Design review of the part built by this model. Coordinates are the model's own, in mm. A direction names the side the tool comes from. Round coordinates to 2 decimals unless told otherwise and drop trailing zeros. Write each loop counter-clockwise with the first axis right and the second up, starting at its lowest first coordinate (ties: lowest second). Pieces come first, ordered by that corner, then holes. Notation, with made-up numbers: (-17, 37) - (4, 37) arc R21 cw to (4, 60) - close; hole circle Ø4 at (58, 76.5). An arc over 180 degrees is marked (long way). Use one line per item in the form item = value.
```python
from build123d import *

# Parameters (mm, degrees)
F0_W     = 609.6
F0_H     = 609.6
F1_DEPTH = 4.7625
F2_W     = 193.675
F2_H     = 193.675
F2_W_2   = 184.15
F2_H_2   = 184.15
F3_DEPTH = 152.4
F4_R     = 3.175
F5_DEPTH = 25.4
F6_R     = 3.175
F7_DEPTH = 401.6385
F8_R     = 3.175
F9_DEPTH = 401.6385


with BuildPart() as f1:
    # F0 (on Top) → F1 (new body)
    with BuildSketch(Plane.XY):
        with Locations((-304.8, 304.8)):
            Rectangle(F0_W, F0_H)
    extrude(amount=F1_DEPTH)

    # F2 (on face) → F3 (join)
    with BuildSketch(Plane.XY.offset(4.7625)):
        with Locations((-304.8, 304.8)):
            Rectangle(F2_W, F2_H)
        with Locations((-304.8, 304.8)):
            Rectangle(F2_W_2, F2_H_2, mode=Mode.SUBTRACT)
    extrude(amount=F3_DEPTH)

    # F4 (on face) → F5 (cut)
    with BuildSketch(Plane.XY.offset(4.7625)):
        with Locations((-25.4, 584.2)):
            Circle(F4_R)
        with Locations((-25.4, 25.4)):
            Circle(F4_R)
        with Locations((-584.2, 584.2)):
            Circle(F4_R)
        with Locations((-584.2, 25.4)):
            Circle(F4_R)
        with Locations((-25.4, 406.4)):
            Circle(F4_R)
        with Locations((-25.4, 203.2)):
            Circle(F4_R)
        with Locations((-584.2, 406.4)):
            Circle(F4_R)
        with Locations((-584.2, 203.2)):
            Circle(F4_R)
        with Locations((-406.4, 25.4)):
            Circle(F4_R)
        with Locations((-406.4, 584.2)):
            Circle(F4_R)
        with Locations((-203.2, 25.4)):
            Circle(F4_R)
        with Locations((-203.2, 584.2)):
            Circle(F4_R)
    extrude(amount=-F5_DEPTH, mode=Mode.SUBTRACT)

    # F6 (on face) → F7 (cut, through all)
    with BuildSketch(Plane.XZ.offset(-207.9625)):
        with Locations((-350.8375, 119.0625)):
            Circle(F6_R)
        with Locations((-258.7625, 119.0625)):
            Circle(F6_R)
    extrude(amount=-F7_DEPTH, mode=Mode.SUBTRACT)

    # F8 (on face) → F9 (cut, through all)
    with BuildSketch(Plane(origin=(-401.6375, 0, 0), x_dir=(0, -1, 0), z_dir=(-1, 0, 0))):
        with Locations((-258.7625, 93.6625)):
            Circle(F8_R)
        with Locations((-350.8375, 93.6625)):
            Circle(F8_R)
    extrude(amount=-F9_DEPTH, mode=Mode.SUBTRACT)


solid = f1.part
```
Q1. We need section B-B on z = 31. Write out the cut boundary in (x, y) (1 decimal).
Calculated:
outline = (-401.6, 208) - (-208, 208) - (-208, 401.6) - (-401.6, 401.6) - close; hole (-396.9, 212.7) - (-212.7, 212.7) - (-212.7, 396.9) - (-396.9, 396.9) - close
Q2. We need section A-A on y = 242. Write out the cut boundary in (x, z) (1 decimal), then the cut area to 3 significant figures.
Calculated:
outline = (-609.6, 0) - (0, 0) - (0, 4.8) - (-208, 4.8) - (-208, 157.2) - (-212.7, 157.2) - (-212.7, 4.8) - (-396.9, 4.8) - (-396.9, 157.2) - (-401.6, 157.2) - (-401.6, 4.8) - (-609.6, 4.8) - close
area = 4,350 mm2
Q3. Draft analysis for pull direction Y (two halves, no side actions). For faces 6 (the flat face through (-306, 207.962, 80)), 7 (the flat face through (-445, 309, 4.762)), 8 (the flat face through (-212.725, 304, 80)), state which applies: released by +Y, released by -Y, zero draft, split by the parting line, or undercut.
Calculated:
face_6 = released by -Y
face_7 = zero draft
face_8 = undercut
Q4. Machinability: for faces 1 (the flat face through (-306, 401.638, 80)), 2 (the flat face through (-309, 309, 0)), 3 (the flat face through (-306, 306, 4.762)), 4 (the flat face through (-207.962, 303, 80)), 5 (the flat face through (-401.638, 303, 80)), which of the approach directions +Z, -Z, +X, -X, +Y, -Y give a long, thin tool a straight path to every point of the face, cutting with its end or side? Answer none if there is none.
Calculated:
face_1 = +Z, +X, -X, +Y
face_2 = -Z, +X, -X, +Y, -Y
face_3 = +Z
face_4 = +Z, +X, +Y, -Y
face_5 = +Z, -X, +Y, -Y
Q5. For P1, Ø8, axis at y = 360, z = 42.5, coming from the -X side; P2, Ø1.5, axis at x = -268.5, z = 130.5, coming from the +Y side; P3, Ø7.5, axis at x = -25.4, y = 584.2, coming from the +Z side; P4, Ø10, axis at x = -477.5, y = 441, coming from the -Z side, all flat-tipped, find the tip position at first contact; note any pin that passes through.
Calculated:
P1 = -401.64
P2 = 401.64
P3 = 4.76
P4 = 0
Q6. We need section C-C on x = -560.5. Write out the cut boundary in (y, z), then the cut area to 3 significant figures.
Calculated:
outline = (0, 0) - (609.6, 0) - (609.6, 4.76) - (0, 4.76) - close
area = 2,900 mm2
Q7. We need section D-D on y = 120.5. Write out the cut boundary in (x, z).
Calculated:
outline = (-609.6, 0) - (0, 0) - (0, 4.76) - (-609.6, 4.76) - close
Q8. To check wall thickness, follow line 1 along X through (y, z) = (584.2, 3.5) (3 decimals); line 2 along X through (y, z) = (25, 2); line 3 along Y through (x, z) = (-25.4, 1.9) (3 decimals). State the ranges of each line that lie inside material, in increasing order. Write a range as from..to.
Calculated:
line_1 = -609.6..-587.375, -581.025..-409.575, -403.225..-206.375, -200.025..-28.575, -22.225..0
line_2 = -609.6..-587.35, -581.05..-409.55, -403.25..-206.35, -200.05..-28.55, -22.25..0
line_3 = 0..22.225, 28.575..200.025, 206.375..403.225, 409.575..581.025, 587.375..609.6
